Could you check a few things on this model? Use its own coordinates, in mm. A direction names the side the tool comes from. Coordinates: 2 decimals unless noted, no trailing zeros. Loops run counter-clockwise (first coordinate to the right, second up) from the corner with the lowest first, then second, coordinate; pieces in that order, holes last. Notation, with made-up numbers: M 66.25,-8.5 L 83.25,-8.5 A6 ccw 83.25,-0.5 Z; hole C -0.75,53 d2. An arc over 180 degrees is marked long. Use one line per item in the form item = value. Start each with the question number.
```python
from build123d import *

# Parameters (mm, degrees)
BOSS_EXTRUDE1_DEPTH = 15
SKETCH2_R           = 1
CUT_EXTRUDE1_DEPTH  = 4
SKETCH3_R           = 1
CUT_EXTRUDE2_DEPTH  = 4


with BuildPart() as part:
    # Sketch1 → Boss-Extrude1 (new body)
    with BuildSketch(Plane.XY):
        with BuildLine():
            ThreePointArc((1.5, 0), (0, 1.5), (-1.5, 0))
            ThreePointArc((-1.5, 0), (-0.714591942, -2.739389257), (-1.5, -5.478778514))
            ThreePointArc((-1.5, -5.478778514), (0, -6.978778514), (1.5, -5.478778514))
            ThreePointArc((1.5, -5.478778514), (0.714591942, -2.739389257), (1.5, 0))
        make_face()
    extrude(amount=BOSS_EXTRUDE1_DEPTH)

    # Sketch2 → Cut-Extrude1 (cut)
    with BuildSketch(Plane.XY.offset(15)):
        with Locations((0, 0.2)):
            Circle(SKETCH2_R)
        with Locations((0, -5.678778514)):
            Circle(SKETCH2_R)
    extrude(amount=-CUT_EXTRUDE1_DEPTH, mode=Mode.SUBTRACT)

    # Sketch3 → Cut-Extrude2 (cut)
    with BuildSketch(Plane(origin=(0, 0, 0), x_dir=(-1, 0, 0), z_dir=(0, 0, -1))):
        with Locations((0, 0.2)):
            Circle(SKETCH3_R)
        with Locations((0, -5.678778514)):
            Circle(SKETCH3_R)
    extrude(amount=-CUT_EXTRUDE2_DEPTH, mode=Mode.SUBTRACT)


solid = part.part
```
Item 1: I want a section at B-B (y = -0.5). Write out the boundary of the cut face in (x, z), plus the area to 3 significant figures.
Item 2: Thinking about a two-plate mould opening in Y: for faces 1 (the cylindrical face through (0.217, -0.776, 1.972)), 2 (the cylindrical face through (0, 1.5, 7.4)), 3 (the flat face through (0, 0, 4)), 4 (the flat face through (0, -3, 0)), which applies, pulls with the +Y half, pulls with the -Y half, needs draft (parallel to the pull), parting line crosses it, or undercut?
Item 3: I want a section at A-A (z = 1.25). Write out the boundary of the cut face in (x, y), plus the area to 3 significant figures.
Item 4: I want a section at C-C (x = -0.55). Write out the boundary of the cut face in (y, z).
Item 5: I want a section at D-D (z = 7.25). Write out the boundary of the cut face in (x, y).
Item 6: For faces 5 (the cylindrical face through (-0.03, -6.98, 7.4)), 6 (the flat face through (0, 0, 11)), 7 (the flat face through (0, -6, 4)), which set-ups out of +Z, -Z, +X, -X, +Y, -Y let a thin tool reach every point of the face, with its end or its side?
Item 7: Please list where these lines run through material, in increasing order: line 1 along Y through (x, z) = (0, 12.15); line 2 along Y through (x, z) = (-0.4, 14.25); line 3 along Z through (x, y) = (0.15, -6).
Item 8: I'm going to push flat-ended pins straight in: P1, Ø0.6, axis at x = 0.5, y = 0.5, coming from the -Z side; P2, Ø1.6, axis at x = 0, y = 0.2, coming from the +Z side. Where does each tip first touch, or does it pass through?
Worked answers:
q1.outline = M -1.22,0 L -0.71,0 L -0.71,4 L 0.71,4 L 0.71,0 L 1.22,0 L 1.22,15 L 0.71,15 L 0.71,11 L -0.71,11 L -0.71,15 L -1.22,15 Z
q1.area = 25.3 mm²
q2.face_1 = undercut
q2.face_2 = pulls with the +Y half
q2.face_3 = undercut
q2.face_4 = needs draft
q3.outline = M -1.5,-5.48 A1.5 ccw 1.5,-5.48 A5.17 cw 1.5,0 A1.5 ccw -1.5,0 A5.17 cw Z; hole C 0,-5.68 d2; hole C 0,0.2 d2
q3.area = 11.4 mm²
q4.outline = M -6.87,0 L -6.51,0 L -6.51,4 L -4.84,4 L -4.84,0 L -0.64,0 L -0.64,4 L 1.04,4 L 1.04,0 L 1.4,0 L 1.4,15 L 1.04,15 L 1.04,11 L -0.64,11 L -0.64,15 L -4.84,15 L -4.84,11 L -6.51,11 L -6.51,15 L -6.87,15 Z
q5.outline = M -1.5,-5.48 A1.5 ccw 1.5,-5.48 A5.17 cw 1.5,0 A1.5 ccw -1.5,0 A5.17 cw Z
q6.face_5 = +Z, -Z, -Y
q6.face_6 = +Z
q6.face_7 = -Z
q7.line_1 = -6.98 to -6.68, -4.68 to -0.8, 1.2 to 1.5
q7.line_2 = -6.92 to -6.6, -4.76 to -0.72, 1.12 to 1.45
q7.line_3 = 4 to 11
q8.P1 = 4
q8.P2 = 11
